Work out the finished part from the listing and answer in its coordinate system (mm). A direction names the side the tool comes from. Coordinates: 2 decimals unless noted, no trailing zeros. Loops run counter-clockwise (first coordinate to the right, second up) from the corner with the lowest first, then second, coordinate; pieces in that order, holes last. Notation, with made-up numbers: (5, 17.25) -> (40, 17.25) arc R26 ccw to (40, 39.25) -> close; hole circle Ø7 at (41, 82.25). An arc over 180 degrees is marked (long way). One line per question, with ' | ' between items.
```python
from build123d import *

# Parameters (mm, degrees)
F0_W     = 76.2
F0_H     = 63.5
F1_DEPTH = 56.896
F2_DEPTH = 25.4


with BuildPart() as f1:
    # F0 (on Right) → F1 (new body)
    with BuildSketch(Plane.YZ):
        Polygon((-61.684637, -50.062766), (39.915363, -49.619449), (39.915363, 26.580551), (-61.684637, 26.580551), align=None)
        with Locations((-10.884637, -11.519449)):
            Rectangle(F0_W, F0_H, mode=Mode.SUBTRACT)
    extrude(amount=F1_DEPTH)

    # F0 (on Right) → F2 (join)
    with BuildSketch(Plane.YZ):
        with Locations((-10.884637, -11.519449)):
            Rectangle(F0_W, F0_H)
    extrude(amount=F2_DEPTH)


solid = f1.part
```
1) Find section B-B (z = -35.5). Write down the section's boundary in (x, y).
Check values:
outline: (0, -61.68) -> (56.9, -61.68) -> (56.9, -48.98) -> (25.4, -48.98) -> (25.4, 27.22) -> (56.9, 27.22) -> (56.9, 39.92) -> (0, 39.92) -> close
2) For faces 1 (the face through (41, -11, -43.269)), 2 (the face through (56.896, -12, -45)), determine the directions among +Z, -Z, +X, -X, +Y, -Y from which every point of the face is accessible in a straight line to the end or side of a thin tool.
Check values:
face 1: +X | face 2: +Z, -Z, +X, +Y, -Y
3) Find section C-C (y = -36). Write down the section's boundary in (x, z).
Check values:
outline: (0, -49.95) -> (56.9, -49.95) -> (56.9, -43.27) -> (25.4, -43.27) -> (25.4, 20.23) -> (56.9, 20.23) -> (56.9, 26.58) -> (0, 26.58) -> close
4) Find section A-A (x = 27). Write down the section's boundary in (y, z), plus the area to 3 significant figures.
Check values:
outline: (-61.68, -50.06) -> (39.92, -49.62) -> (39.92, 26.58) -> (-61.68, 26.58) -> close; hole (-48.98, -43.27) -> (27.22, -43.27) -> (27.22, 20.23) -> (-48.98, 20.23) -> close | area: 2,930 mm^2
5) Flat-ended cylindrical pins translate along their axes: pin 1 (1.5 mm diameter, centred on x = 41.5, y = -45.5, fed in from -Z); pin 2 (4 mm diameter, centred on y = -40.5, z = 5, fed in from +X); pin 3 (1 mm diameter, centred on x = 11.5, y = 15, fed in from -Z). Find the tip coordinate at first contact, or state that the pin passes through.
Check values:
pin 1: stops at z = -50 | pin 2: stops at x = 25.4 | pin 3: stops at z = -49.73
6) The mould has two halves that part along Z. Classify faces 3 (the face through (41, -48.985, -12)), 4 (the face through (28, -10, 26.581)), 5 (the face through (0, -12, -11)): released by +Z, released by -Z, zero draft, split by the parting line, or undercut.
Check values:
face 3: undercut | face 4: released by +Z | face 5: zero draft
7) Find the intervals of material crossed by line 1 along Y through (x, z) = (35, -31); line 2 along X through (y, z) = (-48, -34.5); line 3 along Z through (x, y) = (25.5, -10), in increasing order.
Check values:
line 1: y = -61.68 to -48.98, 27.22 to 39.92 | line 2: x = 0 to 25.4 | line 3: z = -49.84 to -43.27, 20.23 to 26.58
